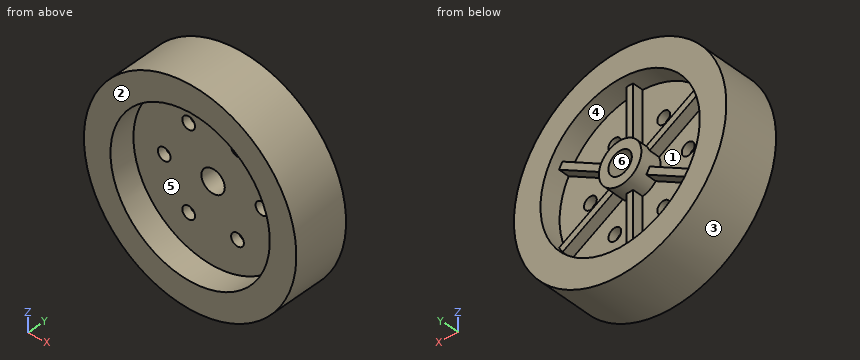
from build123d import *

# Parameters (mm, degrees)
SKETCH1_R           = 50
SKETCH1_R_2         = 37.5
BOSS_EXTRUDE1_DEPTH = 26
BOSS_EXTRUDE3_DEPTH = 9
BOSS_EXTRUDE4_START = -14
SKETCH9_R           = 10
SKETCH9_R_2         = 5.5
BOSS_EXTRUDE4_DEPTH = 14
SKETCH10_R          = 3
BOSS_EXTRUDE5_DEPTH = 4


with BuildPart() as part:
    # Sketch1 → Boss-Extrude1 (new body)
    with BuildSketch(Plane(origin=(0, 0, 0), x_dir=(1, 0, 0), z_dir=(0, 1, 0))):
        with Locations(Location((0, 0, 0), (0, 0, 90))):
            Circle(SKETCH1_R)
        with Locations(Location((0, 0, 0), (0, 0, 90))):
            Circle(SKETCH1_R_2, mode=Mode.SUBTRACT)
    extrude(amount=BOSS_EXTRUDE1_DEPTH)

    # Sketch3 → Boss-Extrude3 (add)
    with BuildSketch(Plane(origin=(0, 12, 0), x_dir=(1, 0, 0), z_dir=(0, 1, 0))):
        with BuildLine():
            Line((1.603162061, 37.465715947), (1.603162061, 9.870657091))
            ThreePointArc((1.603162061, 9.870657091), (0, 10), (-1.603162061, 9.870657091))
            Line((-1.603162061, 9.870657091), (-1.603162061, 37.465715947))
            ThreePointArc((-1.603162061, 37.465715947), (0, 37.5), (1.603162061, 37.465715947))
        make_face()
        with BuildLine():
            Line((31.64468075, 20.121237045), (7.746658762, 6.323707617))
            ThreePointArc((7.746658762, 6.323707617), (8.660254038, 5), (9.349820823, 3.546949474))
            Line((9.349820823, 3.546949474), (33.247842811, 17.344478902))
            ThreePointArc((33.247842811, 17.344478902), (32.475952642, 18.75), (31.64468075, 20.121237045))
        make_face()
        with BuildLine():
            Line((33.247842811, -17.344478902), (9.349820823, -3.546949474))
            ThreePointArc((9.349820823, -3.546949474), (8.660254038, -5), (7.746658762, -6.323707617))
            Line((7.746658762, -6.323707617), (31.64468075, -20.121237045))
            ThreePointArc((31.64468075, -20.121237045), (32.475952642, -18.75), (33.247842811, -17.344478902))
        make_face()
        with BuildLine():
            Line((1.603162061, -37.465715947), (1.603162061, -9.870657091))
            ThreePointArc((1.603162061, -9.870657091), (0, -10), (-1.603162061, -9.870657091))
            Line((-1.603162061, -9.870657091), (-1.603162061, -37.465715947))
            ThreePointArc((-1.603162061, -37.465715947), (0, -37.5), (1.603162061, -37.465715947))
        make_face()
        with BuildLine():
            Line((-31.64468075, -20.121237045), (-7.746658762, -6.323707617))
            ThreePointArc((-7.746658762, -6.323707617), (-8.660254038, -5), (-9.349820823, -3.546949474))
            Line((-9.349820823, -3.546949474), (-33.247842811, -17.344478902))
            ThreePointArc((-33.247842811, -17.344478902), (-32.475952642, -18.75), (-31.64468075, -20.121237045))
        make_face()
        with BuildLine():
            Line((-33.247842811, 17.344478902), (-9.349820823, 3.546949474))
            ThreePointArc((-9.349820823, 3.546949474), (-8.660254038, 5), (-7.746658762, 6.323707617))
            Line((-7.746658762, 6.323707617), (-31.64468075, 20.121237045))
            ThreePointArc((-31.64468075, 20.121237045), (-32.475952642, 18.75), (-33.247842811, 17.344478902))
        make_face()
    extrude(amount=BOSS_EXTRUDE3_DEPTH)

    # Sketch9 → Boss-Extrude4 (add)
    with BuildSketch(Plane(origin=(0, 26, 0), x_dir=(1, 0, 0), z_dir=(0, 1, 0)).offset(BOSS_EXTRUDE4_START)):
        with Locations(Location((0, 0, 0), (0, 0, 270))):
            Circle(SKETCH9_R)
        with Locations(Location((0, 0, 0), (0, 0, 270))):
            Circle(SKETCH9_R_2, mode=Mode.SUBTRACT)
    extrude(amount=BOSS_EXTRUDE4_DEPTH)

    # Sketch10 → Boss-Extrude5 (add)
    # profile 1 of 6: a face of its own
    with BuildSketch(Plane(origin=(0, 12, 0), x_dir=(1, 0, 0), z_dir=(0, 1, 0))):
        with BuildLine():
            Line((7.746658762, 6.323707617), (31.64468075, 20.121237045))
            ThreePointArc((31.64468075, 20.121237045), (18.75, 32.475952642), (1.603162061, 37.465715947))
            Line((1.603162061, 37.465715947), (1.603162061, 9.870657091))
            ThreePointArc((1.603162061, 9.870657091), (5, 8.660254038), (7.746658762, 6.323707617))
        make_face()
        with Locations(Location((11.5, 19.918584287, 0), (0, 0, 270))):
            Circle(SKETCH10_R, mode=Mode.SUBTRACT)
    # profile 2 of 6: a face of its own
    with BuildSketch(Plane(origin=(0, 12, 0), x_dir=(1, 0, 0), z_dir=(0, 1, 0))):
        with BuildLine():
            Line((33.247842811, 17.344478902), (9.349820823, 3.546949474))
            ThreePointArc((9.349820823, 3.546949474), (10, 0), (9.349820823, -3.546949474))
            Line((9.349820823, -3.546949474), (33.247842811, -17.344478902))
            ThreePointArc((33.247842811, -17.344478902), (37.5, 0), (33.247842811, 17.344478902))
        make_face()
        with Locations(Location((23, 0, 0), (0, 0, 270))):
            Circle(SKETCH10_R, mode=Mode.SUBTRACT)
    # profile 3 of 6: a face of its own
    with BuildSketch(Plane(origin=(0, 12, 0), x_dir=(1, 0, 0), z_dir=(0, 1, 0))):
        with BuildLine():
            Line((31.64468075, -20.121237045), (7.746658762, -6.323707617))
            ThreePointArc((7.746658762, -6.323707617), (5, -8.660254038), (1.603162061, -9.870657091))
            Line((1.603162061, -9.870657091), (1.603162061, -37.465715947))
            ThreePointArc((1.603162061, -37.465715947), (18.75, -32.475952642), (31.64468075, -20.121237045))
        make_face()
        with Locations(Location((11.5, -19.918584287, 0), (0, 0, 270))):
            Circle(SKETCH10_R, mode=Mode.SUBTRACT)
    # profile 4 of 6: a face of its own
    with BuildSketch(Plane(origin=(0, 12, 0), x_dir=(1, 0, 0), z_dir=(0, 1, 0))):
        with BuildLine():
            Line((-1.603162061, -37.465715947), (-1.603162061, -9.870657091))
            ThreePointArc((-1.603162061, -9.870657091), (-5, -8.660254038), (-7.746658762, -6.323707617))
            Line((-7.746658762, -6.323707617), (-31.64468075, -20.121237045))
            ThreePointArc((-31.64468075, -20.121237045), (-18.75, -32.475952642), (-1.603162061, -37.465715947))
        make_face()
        with Locations(Location((-11.5, -19.918584287, 0), (0, 0, 270))):
            Circle(SKETCH10_R, mode=Mode.SUBTRACT)
    # profile 5 of 6: a face of its own
    with BuildSketch(Plane(origin=(0, 12, 0), x_dir=(1, 0, 0), z_dir=(0, 1, 0))):
        with BuildLine():
            Line((-33.247842811, -17.344478902), (-9.349820823, -3.546949474))
            ThreePointArc((-9.349820823, -3.546949474), (-10, 0), (-9.349820823, 3.546949474))
            Line((-9.349820823, 3.546949474), (-33.247842811, 17.344478902))
            ThreePointArc((-33.247842811, 17.344478902), (-37.5, 0), (-33.247842811, -17.344478902))
        make_face()
        with Locations(Location((-23, 0, 0), (0, 0, 270))):
            Circle(SKETCH10_R, mode=Mode.SUBTRACT)
    # profile 6 of 6: a face of its own
    with BuildSketch(Plane(origin=(0, 12, 0), x_dir=(1, 0, 0), z_dir=(0, 1, 0))):
        with BuildLine():
            Line((-31.64468075, 20.121237045), (-7.746658762, 6.323707617))
            ThreePointArc((-7.746658762, 6.323707617), (-5, 8.660254038), (-1.603162061, 9.870657091))
            Line((-1.603162061, 9.870657091), (-1.603162061, 37.465715947))
            ThreePointArc((-1.603162061, 37.465715947), (-18.75, 32.475952642), (-31.64468075, 20.121237045))
        make_face()
        with Locations(Location((-11.5, 19.918584287, 0), (0, 0, 270))):
            Circle(SKETCH10_R, mode=Mode.SUBTRACT)
    extrude(amount=BOSS_EXTRUDE5_DEPTH)


solid = part.part
The model under review builds one solid part; all positions refer to its coordinate system, in mm. Face numbers are marked on the shaded views. A direction names the side the tool comes from. Coordinates: 2 decimals unless noted, no trailing zeros. Loops run counter-clockwise (first coordinate to the right, second up) from the corner with the lowest first, then second, coordinate; pieces in that order, holes last.
(1) Draft analysis for pull direction Z (two halves, no side actions). For the marked faces 1, 2 and 3, state which applies: +Z half, -Z half, draft (parallel to the pull), parting line (faces both ways), or undercut.
Determined:
face 1: undercut
face 2: draft
face 3: parting line
(2) Tool access review of the marked faces 4, 5 and 6: name each direction out of +Z, -Z, +X, -X, +Y, -Y from which nothing blocks a thin tool from reaching the whole face with its end or side.
Determined:
face 4: +Y
face 5: -Y
face 6: +Y, -Y
(3) Consider section B-B, the plane y = 14. Give the boundary of the cut face in (x, z).
Determined:
outline: circle Ø100 at (0, 0); hole circle Ø6 at (-23, 0); hole circle Ø6 at (-11.5, -19.92); hole circle Ø6 at (-11.5, 19.92); hole circle Ø11 at (0, 0); hole circle Ø6 at (11.5, -19.92); hole circle Ø6 at (11.5, 19.92); hole circle Ø6 at (23, 0)
(4) Consider section C-C, the plane x = 0. Give the boundary of the cut face in (y, z).
Determined:
outline: (0, -50) - (26, -50) - (26, -37.5) - (21, -37.5) - (21, -10) - (26, -10) - (26, -5.5) - (12, -5.5) - (12, -37.5) - (0, -37.5) - close; (0, 37.5) - (12, 37.5) - (12, 5.5) - (26, 5.5) - (26, 10) - (21, 10) - (21, 37.5) - (26, 37.5) - (26, 50) - (0, 50) - close
(5) Consider section A-A, the plane z = 0. Give the boundary of the cut face in (x, y), plus the area to 3 significant figures.
Determined:
outline: (-50, 0) - (-37.5, 0) - (-37.5, 12) - (-26, 12) - (-26, 16) - (-37.5, 16) - (-37.5, 26) - (-50, 26) - close; (-20, 12) - (-5.5, 12) - (-5.5, 26) - (-10, 26) - (-10, 16) - (-20, 16) - close; (5.5, 12) - (20, 12) - (20, 16) - (10, 16) - (10, 26) - (5.5, 26) - close; (26, 12) - (37.5, 12) - (37.5, 0) - (50, 0) - (50, 26) - (37.5, 26) - (37.5, 16) - (26, 16) - close
area: 948 mm2
(6) Wall thickness on L1, parallel to X at y = 23.25, z = 4; L2, parallel to Z at x = 0.5, y = 16; L3, parallel to X at y = 20.5, z = -34.5: over which ranges is each line inside the solid? List them lowest first.
Determined:
L1: x = -49.84 to -37.29, -9.17 to -3.77, 3.77 to 9.17, 37.29 to 49.84
L2: z = -50 to -5.48, 5.48 to 50
L3: x = -36.19 to -14.7, -1.6 to 1.6, 14.7 to 36.19
(7) Insertion check: P1, Ø3.5, axis at x = 0, z = -26.5, coming from the +Y side; P2, Ø12, axis at y = 20.5, z = -17.5, coming from the -X side; P3, Ø2.5, axis at y = 19, z = 28, coming from the -X side. Each pin has a flat end and moves straight along its axis. Give the tip position at first contact, or say it passes through.
Determined:
P1: stops at y = 21
P2: stops at x = -48.66
P3: stops at x = -42.24
(8) Consider section D-D, the plane x = -11.5. Give the boundary of the cut face in (y, z), plus the area to 3 significant figures.
Determined:
outline: (0, -48.66) - (26, -48.66) - (26, -35.69) - (16, -35.69) - (16, -22.92) - (12, -22.92) - (12, -35.69) - (0, -35.69) - close; (0, 35.69) - (12, 35.69) - (12, 22.92) - (16, 22.92) - (16, 35.69) - (26, 35.69) - (26, 48.66) - (0, 48.66) - close; (12, -16.92) - (16, -16.92) - (16, -8.49) - (21, -8.49) - (21, -4.79) - (16, -4.79) - (16, 4.79) - (21, 4.79) - (21, 8.49) - (16, 8.49) - (16, 16.92) - (12, 16.92) - close
area: 949 mm2
